```python
from build123d import *

# Parameters (mm, degrees)
F0_W     = 200
F0_H     = 20
F1_DEPTH = 40
F2_W     = 10
F2_H     = 40
F3_DEPTH = 10
F4_DEPTH = 15
F5_W     = 10
F5_H     = 3
F6_DEPTH = 10
F7_W     = 10
F7_H     = 3.26613
F8_DEPTH = 10


with BuildPart() as f1:
    # F0 (on Front) → F1 (new body)
    with BuildSketch(Plane.XZ):
        Rectangle(F0_W, F0_H)
    extrude(amount=F1_DEPTH)

    # F2 (on face) → F3 (join)
    with BuildSketch(Plane.XY.offset(10)):
        with Locations((64.525982, -20)):
            Rectangle(F2_W, F2_H)
    extrude(amount=F3_DEPTH)

    # F2 (on face) → F4 (join)
    with BuildSketch(Plane.XY.offset(10)):
        with Locations((64.525982, -20)):
            Rectangle(F2_W, F2_H)
        with Locations((-46.073499, -20)):
            Rectangle(F2_W, F2_H)
    extrude(amount=F4_DEPTH)

    # F5 (on face) → F6 (cut)
    with BuildSketch(Plane.XY.offset(25)):
        with Locations((-46.073499, -20)):
            Rectangle(F5_W, F5_H)
    extrude(amount=-F6_DEPTH, mode=Mode.SUBTRACT)

    # F7 (on face) → F8 (cut)
    with BuildSketch(Plane.XY.offset(25)):
        with Locations((64.525982, -20.022178)):
            Rectangle(F7_W, F7_H)
    extrude(amount=-F8_DEPTH, mode=Mode.SUBTRACT)


solid = f1.part
```
Design review of the part built by this model. Coordinates are the model's own, in mm. A direction names the side the tool comes from. Round coordinates to 2 decimals unless told otherwise and drop trailing zeros. Order: outer loops, then holes, each group sorted by start corner. A loop starts at its lowest first (then second) coordinate and runs counter-clockwise, first axis right, second up. Notation, with made-up numbers: (-0.5, -3.5) - (7.5, -3.5) arc R23 cw to (7.5, 34.5) - close; hole circle Ø9 at (-7.75, 60.25). An arc over 180 degrees is marked (long way). One line per question, with ' | ' between items.
Item 1: Take a section at A-A, the plane z = 12. Write out the cut boundary in (x, y), then the cut area to 3 significant figures.
Checks:
outline: (-51.07, -40) - (-41.07, -40) - (-41.07, 0) - (-51.07, 0) - close; (59.53, -40) - (69.53, -40) - (69.53, 0) - (59.53, 0) - close | area: 800 mm²
Item 2: For P1, Ø7.5, axis at y = -20, z = 16, coming from the +X side; P2, Ø12, axis at y = -35.5, z = 19, coming from the -X side; P3, Ø15, axis at x = 91.5, y = -10, coming from the +Z side; P4, Ø3, axis at x = -48.5, z = 21.5, coming from the +Y side, all flat-tipped, find the tip position at first contact; note any pin that passes through.
Checks:
P1: x = 69.53 | P2: x = -51.07 | P3: z = 10 | P4: y = 0
Item 3: Draft analysis for pull direction X (two halves, no side actions). For faces 6 (the face through (69.526, -20, 14)), 7 (the face through (59.526, -20, 14)), 8 (the face through (-100, -20, 0)), 9 (the face through (-1, -40, 4)), state which applies: +X half, -X half, draft (parallel to the pull), parting line (faces both ways), or undercut.
Checks:
face 6: +X half | face 7: undercut | face 8: -X half | face 9: draft
Item 4: Take a section at C-C, the plane z = 20.5. Write out the cut boundary in (x, y), then the cut area to 3 significant figures.
Checks:
outline: (-51.07, -40) - (-41.07, -40) - (-41.07, -21.5) - (-51.07, -21.5) - close; (-51.07, -18.5) - (-41.07, -18.5) - (-41.07, 0) - (-51.07, 0) - close; (59.53, -40) - (69.53, -40) - (69.53, -21.66) - (59.53, -21.66) - close; (59.53, -18.39) - (69.53, -18.39) - (69.53, 0) - (59.53, 0) - close | area: 737 mm²
Item 5: Wall thickness on line 1 (X direction, y = -29, z = 20); line 2 (Z direction, x = -18.5, y = -35.5): over which ranges is each line inside the solid? List them lowest first. Write a range as [from, to].
Checks:
line 1: [-51.07, -41.07], [59.53, 69.53] | line 2: [-10, 10]
Item 6: Machinability: for faces 1 (the face through (-51.073, -20, 14)), 2 (the face through (-41.073, -20, 14)), 3 (the face through (-46, -18.5, 20)), 4 (the face through (85, -20, 10)), 5 (the face through (64, -21.655, 20)), which of the approach directions +Z, -Z, +X, -X, +Y, -Y give a long, thin tool a straight path to every point of the face, cutting with its end or side? Answer none if there is none.
Checks:
face 1: +Z, -X, +Y, -Y | face 2: +Z, +Y, -Y | face 3: +Z, +X, -X | face 4: +Z, +X, +Y, -Y | face 5: +Z, +X
Item 7: Take a section at D-D, the plane x = 67.5. Write out the cut boundary in (y, z).
Checks:
outline: (-40, -10) - (0, -10) - (0, 25) - (-18.39, 25) - (-18.39, 15) - (-21.66, 15) - (-21.66, 25) - (-40, 25) - close
Item 8: Take a section at B-B, the plane y = -9. Write out the cut boundary in (x, z).
Checks:
outline: (-100, -10) - (100, -10) - (100, 10) - (69.53, 10) - (69.53, 25) - (59.53, 25) - (59.53, 10) - (-41.07, 10) - (-41.07, 25) - (-51.07, 25) - (-51.07, 10) - (-100, 10) - close
